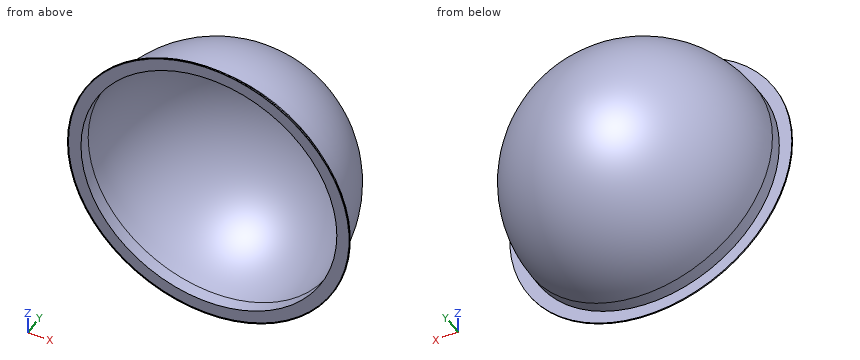
Autodesk Inventor part; units mm, degrees
ref_plane "YZ Plane" through (0, 0, 0) normal (1, 0, 0) x (0, 1, 0)
ref_plane "XZ Plane" through (0, 0, 0) normal (0, 1, 0) x (-1, 0, 0)
ref_plane "XY Plane" through (0, 0, 0) normal (0, 0, 1) x (1, 0, 0)
sketch "Sketch1" plane through (0, 0, 0) normal (0, 1, 0) x (-1, 0, 0)
  circle A0 centre (0, 0) radius 225
  dimension "d0" = 450
extrude "Extrusion1" add sketch "Sketch1" along normal blind 4
sketch "Sketch2" plane through (0, 4, 0) normal (0, 1, 0) x (1, 0, 0)
  circle A0 centre (0, 0) radius 205
  dimension "d3" = 410
extrude "Extrusion2" add sketch "Sketch2" along normal blind 225
sketch "Sketch3" plane through (0, 0, 0) normal (0, -1, 0) x (1, 0, 0)
  circle A0 centre (0, 0) radius 225
  dimension "d7" = 450
extrude "Extrusion3" cut sketch "Sketch3" against normal blind 2
fillet "Fillet2" radius 205 1 edges at (-205, 229, 0)
shell "Shell3" thickness 1 removed faces 1 at (5.0301, 2, -73.6911)
properties part number "450mmdome" material "Polycarbonate, Clear"
The model under review builds one solid part; all positions refer to its coordinate system, in mm. Coordinates: 2 decimals unless noted, no trailing zeros. Loops run counter-clockwise (first coordinate to the right, second up) from the corner with the lowest first, then second, coordinate; pieces in that order, holes last.
(1) Consider section B-B, the plane x = 91. Give the boundary of the cut face in (y, z), plus the area to 3 significant figures.
Determined:
outline: (2, -205.78) - (4, -205.78) - (4, -183.7) - (24, -183.7) arc R183.7 ccw to (24, 183.7) - (4, 183.7) - (4, 205.78) - (2, 205.78) - (2, 204.68) - (3, 204.68) - (3, 182.58) - (24, 182.58) arc R182.58 cw to (24, -182.58) - (3, -182.58) - (3, -204.68) - (2, -204.68) - close
area: 736 mm2
(2) Insertion check: P1, Ø1.5, axis at y = 38.5, z = -132, coming from the -X side; P2, Ø5, axis at y = 37.5, z = 148, coming from the -X side; P3, Ø1, axis at x = 180, z = 101.5, coming from the -Y side. Each pin has a flat end and moves straight along its axis. Give the tip position at first contact, or say it passes through.
Determined:
P1: stops at x = -156.81
P2: stops at x = -143.79
P3: stops at y = 3
(3) Consider section A-A, the plane z = 0. Give the boundary of the cut face in (x, y).
Determined:
outline: (-225, 2) - (-224, 2) - (-224, 3) - (-204, 3) - (-204, 24) arc R204 cw to (204, 24) - (204, 3) - (224, 3) - (224, 2) - (225, 2) - (225, 4) - (205, 4) - (205, 24) arc R205 ccw to (-205, 24) - (-205, 4) - (-225, 4) - close
(4) Wall thickness on L1, parallel to X at y = 10.75, z = 0; L2, parallel to Y at x = 205, z = 52.5: over which ranges is each line inside the solid? List them lowest first.
Determined:
L1: x = -205 to -204, 204 to 205
L2: y = 3 to 4
(5) Consider section C-C, the plane y = 93.5. Give the boundary of the cut face in (x, z), plus the area to 3 significant figures.
Determined:
outline: circle Ø385.72 at (0, 0); hole circle Ø383.59 at (0, 0)
area: 1,280 mm2
